Input: part model. Units: mm. Frame: model coordinates. Give positions to 0.01 mm unless a question says otherwise; leave off trailing zeros. Write each loop counter-clockwise with the first axis right and the second up, starting at its lowest first coordinate (ties: lowest second). Pieces come first, ordered by that corner, then holes. Notation, with made-up numbers: (-35.5, 74) - (22.5, 74) arc R11 cw to (22.5, 95) - close; hole circle Ø8 at (21.5, 65). An arc over 180 degrees is marked (long way). Use a Markdown table: item, result. Add a question column.
1. Mould query, pull axis Z, two halves, no side actions, for faces 1 (the flat face through (-170, 7, 1)), 2 (the cylindrical face through (164.297, 7.395, 113.986)), 3 (the cylindrical face through (-115.95, 7.4, 95.78)). Classes: released by +Z, released by -Z, zero draft, split by the parting line, or undercut.
2. Section query A-A, the plane x = -110. Return loops of the section in (y, z).
3. Section query B-B, the plane z = 95. Return loops of the section in (x, y), plus the area to 3 significant figures.
4. Pin query (flat end, axial travel): pin 1 (11 mm diameter, centred on x = 110, z = 95, fed in from +Y). Return the tip coordinate at first contact, or that it passes through.
5. Material intervals for probe 1 along X at (y, z) = (6.5, 95); probe 2 along X at (y, z) = (7, -93); probe 3 along Z at (x, y) = (-155, 2.25), sorted ascending.
```python
from build123d import *

# Parameters (mm, degrees)
EXTRUDE_1_DEPTH      = 15
SKETCH_2_10_R        = 6
CUT_EXTRUDE_10_DEPTH = 15
SKETCH_2_11_R        = 6
CUT_EXTRUDE_11_DEPTH = 15
SKETCH_2_12_R        = 6
CUT_EXTRUDE_12_DEPTH = 15
SKETCH_2_13_R        = 6
CUT_EXTRUDE_13_DEPTH = 15


with BuildPart() as part:
    # Sketch 2 → Extrude 1 (new body)
    with BuildSketch(Plane(origin=(0, 0, 0), x_dir=(1, 0, 0), z_dir=(0, 1, 0))):
        with BuildLine():
            Line((-150, 120), (150, 120))
            ThreePointArc((150, 120), (164.142135624, 114.142135624), (170, 100))
            Line((170, 100), (170, -100))
            ThreePointArc((170, -100), (164.142135624, -114.142135624), (150, -120))
            Line((150, -120), (-150, -120))
            ThreePointArc((-150, -120), (-164.142135624, -114.142135624), (-170, -100))
            Line((-170, -100), (-170, 100))
            ThreePointArc((-170, 100), (-164.142135624, 114.142135624), (-150, 120))
        make_face()
    extrude(amount=EXTRUDE_1_DEPTH)

    # Sketch 2_10 → Cut-Extrude 10 (cut)
    with BuildSketch(Plane(origin=(0, 0, 0), x_dir=(1, 0, 0), z_dir=(0, 1, 0))):
        with Locations(Location((-110, -95, 0), (0, 0, 90))):
            Circle(SKETCH_2_10_R)
    extrude(amount=CUT_EXTRUDE_10_DEPTH, mode=Mode.SUBTRACT)

    # Sketch 2_11 → Cut-Extrude 11 (cut)
    with BuildSketch(Plane(origin=(0, 0, 0), x_dir=(1, 0, 0), z_dir=(0, 1, 0))):
        with Locations(Location((110, -95, 0), (0, 0, 90))):
            Circle(SKETCH_2_11_R)
    extrude(amount=CUT_EXTRUDE_11_DEPTH, mode=Mode.SUBTRACT)

    # Sketch 2_12 → Cut-Extrude 12 (cut)
    with BuildSketch(Plane(origin=(0, 0, 0), x_dir=(1, 0, 0), z_dir=(0, 1, 0))):
        with Locations(Location((-110, 95, 0), (0, 0, 270))):
            Circle(SKETCH_2_12_R)
    extrude(amount=CUT_EXTRUDE_12_DEPTH, mode=Mode.SUBTRACT)

    # Sketch 2_13 → Cut-Extrude 13 (cut)
    with BuildSketch(Plane(origin=(0, 0, 0), x_dir=(1, 0, 0), z_dir=(0, 1, 0))):
        with Locations(Location((110, 95, 0), (0, 0, 90))):
            Circle(SKETCH_2_13_R)
    extrude(amount=CUT_EXTRUDE_13_DEPTH, mode=Mode.SUBTRACT)


solid = part.part
```
Result sheet:
| question | item | result |
|---|---|---|
| 1 | face 1 | zero draft |
| 1 | face 2 | released by +Z |
| 1 | face 3 | undercut |
| 2 | outline | (0, -120) - (15, -120) - (15, -101) - (0, -101) - close; (0, -89) - (15, -89) - (15, 89) - (0, 89) - close; (0, 101) - (15, 101) - (15, 120) - (0, 120) - close |
| 3 | outline | (-170, 0) - (-116, 0) - (-116, 15) - (-170, 15) - close; (-104, 0) - (104, 0) - (104, 15) - (-104, 15) - close; (116, 0) - (170, 0) - (170, 15) - (116, 15) - close |
| 3 | area | 4,740 mm² |
| 4 | pin 1 | passes through |
| 5 | probe 1 | x = -170 to -116, -104 to 104, 116 to 170 |
| 5 | probe 2 | x = -170 to -115.66, -104.34 to 104.34, 115.66 to 170 |
| 5 | probe 3 | z = -119.36 to 119.36 |
